Design review of the part shown in the three views and the two pictorial views. Dimensions are in mm from the part's minimum x, y and z. A direction names the side the tool comes from. Give positions to 0.01 mm unless a question says otherwise; leave off trailing zeros. Loops run counter-clockwise (first coordinate to the right, second up) from the corner with the lowest first, then second, coordinate; pieces in that order, holes last. Notation, with made-up numbers: (34, 15) - (90, 15) arc R23 ccw to (90, 24) - close; hole circle Ø1 at (-1, -38). An arc over 180 degrees is marked (long way). Answer in a Markdown table with one row per item.
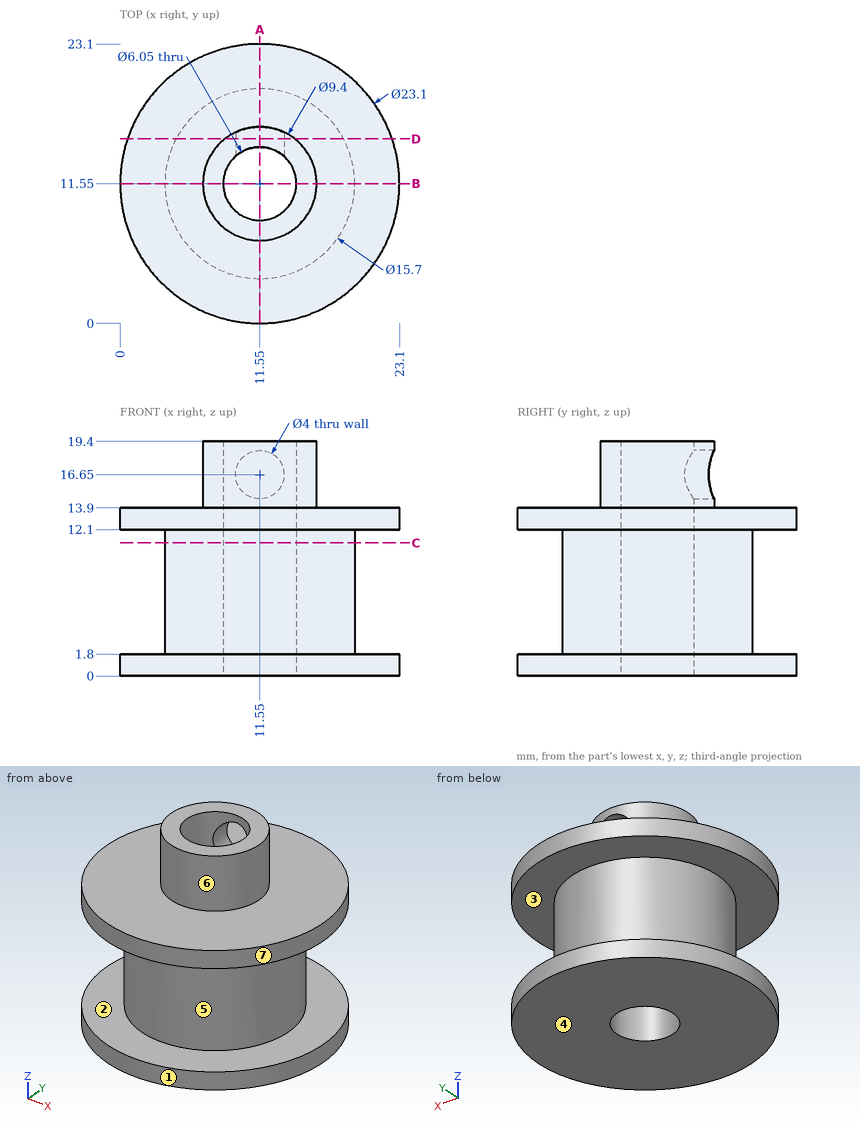
1. Clearance check with flat-ended pins moving along their axes: pin 1 (3 mm diameter, centred on y = 16, z = 14.5, fed in from +X); pin 2 (1 mm diameter, centred on y = 11, z = 17, fed in from +X); pin 3 (5 mm diameter, centred on y = 19.5, z = 5.5, fed in from -X). State where each tip first meets the part, or that it passes through.
Values:
| item | result |
|---|---|
| pin 1 | stops at x = 22.68 |
| pin 2 | stops at x = 16.25 |
| pin 3 | stops at x = 5.9 |
2. For the marked faces 5, 6 and 7, list the 3-axis set-ups (+Z, -Z, +X, -X, +Y, -Y) from which the entire face can be reached by the end or side of a thin tool; tool diameter is ignored.
Values:
| item | result |
|---|---|
| face 5 | none |
| face 6 | +Z |
| face 7 | +Z, -Z |
3. Wall thickness on line 1 (Y direction, x = 11.55, z = 13) (3 decimals); line 2 (Z direction, x = 11.55, y = 15.5); line 3 (Y direction, x = 11.55, z = 6) (3 decimals): over which ranges is each line inside the solid? List them lowest first. Write a range as [from, to].
Values:
| item | result |
|---|---|
| line 1 | y = [0, 8.525], [14.575, 23.1] |
| line 2 | z = [0, 14.65], [18.65, 19.4] |
| line 3 | y = [3.7, 8.525], [14.575, 19.4] |
4. We need section C-C, the plane z = 11. Give the boundary of the cut face in (x, y) (3 decimals), and give its area (3 significant figures).
Values:
| item | result |
|---|---|
| outline | circle Ø15.7 at (11.55, 11.55); hole circle Ø6.05 at (11.55, 11.55) |
| area | 165 mm^2 |
5. We need section A-A, the plane x = 11.55. Give the boundary of the cut face in (y, z) (3 decimals), and give its area (4 significant figures).
Values:
| item | result |
|---|---|
| outline | (0, 0) - (8.525, 0) - (8.525, 19.4) - (6.85, 19.4) - (6.85, 13.9) - (0, 13.9) - (0, 12.1) - (3.7, 12.1) - (3.7, 1.8) - (0, 1.8) - close; (14.575, 0) - (23.1, 0) - (23.1, 1.8) - (19.4, 1.8) - (19.4, 12.1) - (23.1, 12.1) - (23.1, 13.9) - (16.25, 13.9) - (16.25, 14.65) - (14.575, 14.65) - close; (14.575, 18.65) - (16.25, 18.65) - (16.25, 19.4) - (14.575, 19.4) - close |
| area | 172.5 mm^2 |
6. We need section D-D, the plane y = 15.25. Give the boundary of the cut face in (x, z).
Values:
| item | result |
|---|---|
| outline | (0.61, 0) - (22.49, 0) - (22.49, 1.8) - (18.47, 1.8) - (18.47, 12.1) - (22.49, 12.1) - (22.49, 13.9) - (14.45, 13.9) - (14.45, 19.4) - (8.65, 19.4) - (8.65, 13.9) - (0.61, 13.9) - (0.61, 12.1) - (4.63, 12.1) - (4.63, 1.8) - (0.61, 1.8) - close; hole circle Ø4 at (11.55, 16.65) |
7. We need section B-B, the plane y = 11.55. Give the boundary of the cut face in (x, z) (3 decimals).
Values:
| item | result |
|---|---|
| outline | (0, 0) - (8.525, 0) - (8.525, 19.4) - (6.85, 19.4) - (6.85, 13.9) - (0, 13.9) - (0, 12.1) - (3.7, 12.1) - (3.7, 1.8) - (0, 1.8) - close; (14.575, 0) - (23.1, 0) - (23.1, 1.8) - (19.4, 1.8) - (19.4, 12.1) - (23.1, 12.1) - (23.1, 13.9) - (16.25, 13.9) - (16.25, 19.4) - (14.575, 19.4) - close |
8. Mouldability with a two-part tool opening along Z and no side actions: class the marked faces 1, 2, 3 and 4 as released by +Z, released by -Z, zero draft, split by the parting line, or undercut.
Values:
| item | result |
|---|---|
| face 1 | zero draft |
| face 2 | undercut |
| face 3 | undercut |
| face 4 | released by -Z |
